Autodesk Inventor part; units mm, degrees
ref_plane "YZ Plane" through (0, 0, 0) normal (1, 0, 0) x (0, 1, 0)
ref_plane "XZ Plane" through (0, 0, 0) normal (0, 1, 0) x (-1, 0, 0)
ref_plane "XY Plane" through (0, 0, 0) normal (0, 0, 1) x (1, 0, 0)
sketch "Sketch1" plane through (0, 0, 0) normal (1, 0, 0) x (0, 1, 0)
  line L0 (34.6, 0) -> (0, 0)
  line L1 (0, 0) -> (0, -40)
  line L2 (7, -40) -> (7, -5)
  line L3 (7, -5) -> (34.6, -5)
  line L4 (34.6, -5) -> (34.6, 0)
  line L5 (7, -40) -> (0, -40)
  dimension "d0" = 0
  dimension "d1" = 0
  dimension "d2" = 5
  dimension "d3" = 7
  dimension "d5" = 40
  dimension "d6" = 34.6
extrude "Extrusion1" add sketch "Sketch1" along normal blind 16.3
sketch "Sketch2" plane through (0, 7, -5) normal (0, 1, 0) x (1, 0, 0)
  circle A0 centre (8.15, 20) radius 1.5
  line L0 (16.3, 35) -> (16.3, 0)
  line L1 (0, -5) -> (16.3, -5)
  circle A1 centre (8.15, 28) radius 1.5
  line L2 (8.15, 20) -> (8.15, 28) construction
  dimension "d9" = 8.15
  dimension "d10" = 25
  dimension "d11" = 3
  dimension "d31" = 3
  dimension "d32" = 8
extrude "Extrusion2" cut sketch "Sketch2" against normal through all
sketch "Sketch3" plane through (0, 7, -5) normal (0, 0, -1) x (-1, 0, 0)
  line L0 (0, 0) -> (-16.3, 0)
  line L1 (-14.4, 0) -> (-1.9, 0)
  line L2 (-1.9, 0) -> (-1.9, 23)
  line L3 (-1.9, 23) -> (-14.4, 23)
  line L4 (-14.4, 23) -> (-14.4, 0)
  line L5 (0, 0) -> (0, 27.6)
  point P0 (0, -7)
  dimension "d14" = 23
  dimension "d15" = 12.5
  dimension "d16" = 1.9
extrude "Extrusion3" cut sketch "Sketch3" against normal blind 16.3
sketch "Sketch5" plane through (0, 7, -5) normal (0, 0, -1) x (-1, 0, 0)
  line L0 (0, 27.6) -> (-16.3, 27.6)
  line L1 (-16.3, 27.6) -> (0, 27.6)
  line L2 (0, 27.6) -> (0, 0)
  line L3 (0, 0) -> (-1.9, 0)
  line L4 (-14.4, 23) -> (-14.4, 0)
  line L5 (-14.4, 23) -> (-14.4, 0)
  line L6 (-14.4, 0) -> (-16.3, 0)
  line L7 (-16.3, 0) -> (-16.3, 27.6)
  line L8 (-14.4, 23) -> (-1.9, 23)
  line L9 (-1.9, 23) -> (-1.9, 0)
  line L10 (-1.9, 23) -> (-1.9, 0)
  line L11 (-14.4, 23) -> (-1.9, 23)
  point P0 (0, -7)
  dimension "d26" = 0
  dimension "d27" = 0
  dimension "d28" = 1.9
extrude "Extrusion5" add sketch "Sketch5" along normal blind 4
sketch "Sketch4" plane through (0, 0, 0) normal (0, 0, 1) x (1, 0, 0)
  circle A0 centre (8.15, 32.5) radius 1
  circle A1 centre (8.15, 4.5) radius 1
  line L0 (1.9, 30) -> (14.4, 30)
  line L1 (14.4, 7) -> (1.9, 7)
  line L2 (0, 34.6) -> (0, 0)
  line L3 (16.3, 34.6) -> (16.3, 0)
  dimension "d19" = 2.5
  dimension "d20" = 2.5
  dimension "d21" = 2
  dimension "d22" = 8.15
  dimension "d23" = 8.15
extrude "Extrusion4" cut sketch "Sketch4" against normal blind 7
sketch "Sketch6" plane through (0, 7, -40) normal (0, 1, 0) x (1, 0, 0)
  circle A0 centre (12.3, -28) radius 1
  line L0 (0, -40) -> (16.3, -40)
  line L1 (16.3, -40) -> (16.3, -31)
  circle A1 centre (4, -28) radius 1
  line L2 (0, 0) -> (0, -31)
  dimension "d33" = 2
  dimension "d34" = 12
  dimension "d35" = 4
  dimension "d38" = 4
  dimension "d39" = 0
extrude "Extrusion6" cut sketch "Sketch6" against normal blind 10
sketch "Sketch7" plane through (0, 7, -40) normal (0, 1, 0) x (1, 0, 0)
  line L0 (0, 0) -> (0, -31)
  line L1 (0, 0) -> (16.3, 0)
  line L2 (16.3, 0) -> (16.3, -24)
  line L3 (16.3, -24) -> (0, -24)
  line L4 (0, -24) -> (0, 0)
  line L5 (0, -40) -> (16.3, -40)
  line L6 (16.3, 0) -> (16.3, -31)
  point P0 (8.15, -24)
  point P1 (0, -24)
  dimension "d40" = 16
  dimension "d41" = 0
extrude "Extrusion7" cut sketch "Sketch7" against normal blind 10
sketch "Sketch8" plane through (1.9, 7, 0) normal (0, 1, 0) x (1, 0, 0)
  line L0 (14.4, 16) -> (14.4, 9)
  line L1 (-1.9, 0) -> (-1.9, 16)
  line L2 (14.4, 9) -> (-1.9, 9)
  line L3 (-1.9, 9) -> (-1.9, 6)
  line L4 (-1.9, 6) -> (14.4, 6)
  line L5 (14.4, 6) -> (14.4, 9)
  point P0 (-1.9, 9)
  dimension "d44" = 3
extrude "Extrusion8" cut sketch "Sketch8" along normal up to surface (27.6 mm away)
sketch "Sketch9" plane through (1.9, 7, 0) normal (0, 1, 0) x (1, 0, 0)
  circle A0 centre (10.4, 12) radius 1
  circle A1 centre (10.4, 12) radius 3
  circle A2 centre (2.1, 12) radius 1
  circle A3 centre (2.1, 12) radius 3
  point P0 (-1.9, 0)
  dimension "d47" = 6
  dimension "d48" = 6
extrude "Extrusion9" cut sketch "Sketch9" against normal blind 3.5
sketch "Sketch10" plane through (0, 34.6, 0) normal (0, 1, 0) x (1, 0, 0)
  line L0 (0, 0) -> (16.3, 0)
  line L1 (0, 0) -> (0, 16)
  line L2 (16.3, 0) -> (0, 0)
  line L3 (0, 0) -> (0, 0.3)
  line L4 (0, 0.3) -> (16.3, 0.3)
  line L5 (16.3, 0.3) -> (16.3, 0)
  dimension "d51" = 0.3
extrude "Extrusion10" cut sketch "Sketch10" against normal up to surface (34.6 mm away)
sketch "Sketch11" plane through (16.3, 0, 0) normal (1, 0, 0) x (0, 0, -1)
  line L0 (0.3, 0) -> (16, 0)
  line L1 (16, 7) -> (16, 0)
  line L2 (0.3, 0) -> (16, 0)
  line L3 (16, 0) -> (16, 0.3)
  line L4 (16, 0.3) -> (0.3, 0.3)
  line L5 (0.3, 0.3) -> (0.3, 0)
  point P0 (0, 0)
  dimension "d54" = 0.3
extrude "Extrusion11" cut sketch "Sketch11" against normal up to surface (16.3 mm away)
properties part number "ServoHolder_3DPrint"
Design review of the part built by this model. Coordinates are the model's own, in mm. A direction names the side the tool comes from. Round coordinates to 2 decimals unless told otherwise and drop trailing zeros. Loops run counter-clockwise (first coordinate to the right, second up) from the corner with the lowest first, then second, coordinate; pieces in that order, holes last. Notation, with made-up numbers: (77, 56) -> (129, 56) arc R17 ccw to (129, 86) -> close; hole circle Ø5 at (73, 87.25). An arc over 180 degrees is marked (long way). Use one line per item in the form item = value. Start each with the question number.
Q1. We need section A-A on x = 8.15. Give the boundary of the cut face in (y, z), then the cut area to 3 significant figures.
Q2. Wall thickness on line 1 along X through (y, z) = (4.2, -12); line 2 along Y through (x, z) = (8.15, -2.25); line 3 along Z through (x, y) = (12.3, 2.65): over which ranges is each line inside the solid? List them lowest first. Write a range as [from, to].
Q3. We need section D-D on z = -5. Give the boundary of the cut face in (x, y).
Q4. Draft analysis for pull direction Z (two halves, no side actions). For faces 1 (the face through (3, 3.5, -13)), 2 (the face through (8, 4, -16)), 3 (the face through (8, 0.3, -8)), state which applies: +Z half, -Z half, draft (parallel to the pull), parting line (faces both ways), or undercut.
Q5. Machinability: for faces 4 (the face through (8, 7, -8)), 5 (the face through (14, 3.5, -12)), 6 (the face through (14.4, 19, -3)), 7 (the face through (8, 5, -7)), which of the approach directions +Z, -Z, +X, -X, +Y, -Y give a long, thin tool a straight path to every point of the face, cutting with its end or side? Answer none if there is none.
Q6. We need section B-B on z = -12. Give the boundary of the cut face in (x, y).
Q7. For pin 1 Ø7 at (x, z) = (12.3, -12) entering from +Y; pin 2 Ø2.5 at (x, y) = (8.15, 4.5) entering from +Z; pin 3 Ø1 at (x, z) = (10, -12) entering from +Y; pin 4 Ø1.6 at (x, z) = (4, -12) entering from -Y (3 decimals), all flat-tipped, find the tip position at first contact; note any pin that passes through.
Q8. We need section C-C on y = 25.5. Give the boundary of the cut face in (x, z).
Calculated:
q1.outline = (0.3, -16) -> (7, -16) -> (7, -0.3) -> (5.5, -0.3) -> (5.5, -7) -> (3.5, -7) -> (3.5, -0.3) -> (0.3, -0.3) -> close; (30, -6) -> (31.5, -6) -> (31.5, -0.3) -> (30, -0.3) -> close; (33.5, -6) -> (34.6, -6) -> (34.6, -0.3) -> (33.5, -0.3) -> close
q1.area = 107 mm²
q2.line_1 = [0, 1], [7, 9.3], [15.3, 16.3]
q2.line_2 = [0.3, 3.5], [5.5, 7], [30, 31.5], [33.5, 34.6]
q2.line_3 = [-16, -13], [-11, -0.3]
q3.outline = (0, 0.3) -> (16.3, 0.3) -> (16.3, 34.6) -> (0, 34.6) -> close; hole (1.9, 7) -> (14.4, 7) -> (14.4, 30) -> (1.9, 30) -> close; hole circle Ø2 at (8.15, 4.5); hole circle Ø2 at (8.15, 32.5)
q4.face_1 = undercut
q4.face_2 = -Z half
q4.face_3 = draft
q5.face_4 = -Z
q5.face_5 = +Y
q5.face_6 = +Z, -Z
q5.face_7 = +Z
q6.outline = (0, 0.3) -> (3, 0.3) -> (3, 3.5) -> (1, 3.5) -> (1, 7) -> (0, 7) -> close; (5, 0.3) -> (11.3, 0.3) -> (11.3, 3.5) -> (9.3, 3.5) -> (9.3, 7) -> (7, 7) -> (7, 3.5) -> (5, 3.5) -> close; (13.3, 0.3) -> (16.3, 0.3) -> (16.3, 7) -> (15.3, 7) -> (15.3, 3.5) -> (13.3, 3.5) -> close
q7.pin_1 = 7
q7.pin_2 = -0.3
q7.pin_3 = 3.5
q7.pin_4 = through
q8.outline = (0, -6) -> (1.9, -6) -> (1.9, -0.3) -> (0, -0.3) -> close; (14.4, -6) -> (16.3, -6) -> (16.3, -0.3) -> (14.4, -0.3) -> close
